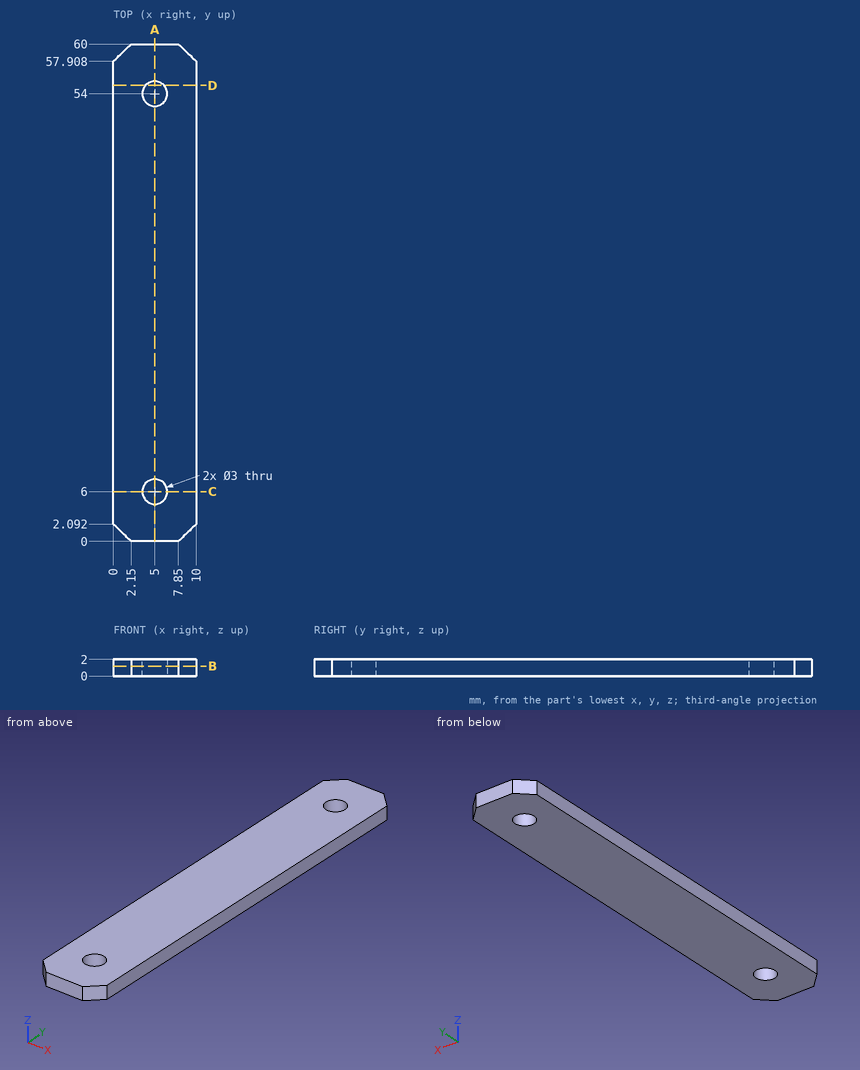
Could you check a few things on this drawing? It's one solid part, dimensions in mm from its lowest x, y, z. Give positions to 0.01 mm unless a question says otherwise; leave off trailing zeros. Order: outer loops, then holes, each group sorted by start corner. A loop starts at its lowest first (then second) coordinate and runs counter-clockwise, first axis right, second up. Notation, with made-up numbers: (-26.75, -38.5) -> (-5.75, -38.5) arc R13 cw to (-5.75, -31.5) -> close; hole circle Ø11 at (-35.5, 64.25). An arc over 180 degrees is marked (long way). Use CSV: the item, a comma, the result in double quotes. Start each with the question number.
Item 1: If I drill on probe 1 along Y at (x, z) = (5, 0.65); probe 2 along Y at (x, z) = (3.75, 0.25); probe 3 along Y at (x, z) = (9.75, 1.1), over which ranges is the centre line in solid material (lowest first)? Write a range as [from, to].
Item 2: Suppose I cut it at A-A (x = 5). List the corners of the cut face in (y, z) for me, and give its area (3 significant figures).
Item 3: Suppose I cut it at C-C (y = 6). List the corners of the cut face in (x, z) for me, and give its area (3 significant figures).
Item 4: Suppose I cut it at D-D (y = 55). List the corners of the cut face in (x, z) for me, and give its area (3 significant figures).
Item 5: Suppose I cut it at B-B (z = 1.2). List the corners of the cut face in (x, y) for me, and give its area (3 significant figures).
Answer block:
1,probe 1,"y = [0, 4.5], [7.5, 52.5], [55.5, 60]"
1,probe 2,"y = [0, 5.17], [6.83, 53.17], [54.83, 60]"
1,probe 3,"y = [1.85, 58.15]"
2,outline,"(0, 0) -> (4.5, 0) -> (4.5, 2) -> (0, 2) -> close; (7.5, 0) -> (52.5, 0) -> (52.5, 2) -> (7.5, 2) -> close; (55.5, 0) -> (60, 0) -> (60, 2) -> (55.5, 2) -> close"
2,area,"108 mm^2"
3,outline,"(0, 0) -> (3.5, 0) -> (3.5, 2) -> (0, 2) -> close; (6.5, 0) -> (10, 0) -> (10, 2) -> (6.5, 2) -> close"
3,area,"14.0 mm^2"
4,outline,"(0, 0) -> (3.88, 0) -> (3.88, 2) -> (0, 2) -> close; (6.12, 0) -> (10, 0) -> (10, 2) -> (6.12, 2) -> close"
4,area,"15.5 mm^2"
5,outline,"(0, 2.09) -> (2.15, 0) -> (7.85, 0) -> (10, 2.09) -> (10, 57.91) -> (7.85, 60) -> (2.15, 60) -> (0, 57.91) -> close; hole circle Ø3 at (5, 6); hole circle Ø3 at (5, 54)"
5,area,"577 mm^2"
